Source: CAD feature listing. Evaluate the final solid. Frame: model axes, mm. Face numbers are marked on the shaded views. A direction names the side the tool comes from. Give positions to 0.01 mm unless a question says otherwise; leave off trailing zeros. Order: outer loops, then holes, each group sorted by start corner. A loop starts at its lowest first (then second) coordinate and runs counter-clockwise, first axis right, second up. Notation, with made-up numbers: (53, 41) - (87, 41) arc R10 ccw to (87, 58) - close; hole circle Ø3 at (2.5, 53.5). An arc over 180 degrees is marked (long way). Answer as CSV lines item,"result".
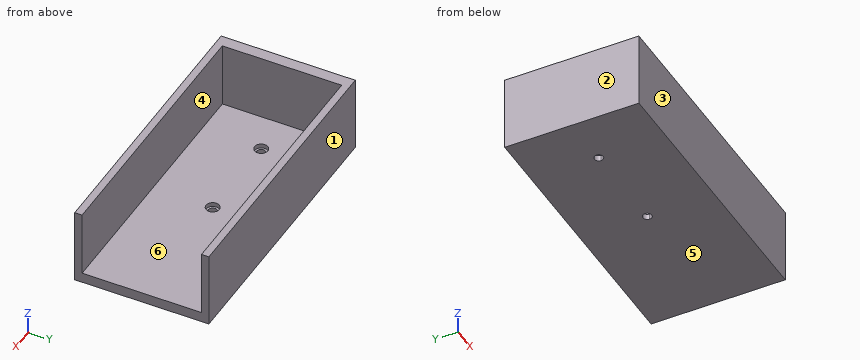
```python
from build123d import *

# Parameters (mm, degrees)
F1_DEPTH = 182
F2_W     = 91
F2_H     = 52
F3_DEPTH = 8
F5_DEPTH = 25
F6_R     = 4.5
F7_DEPTH = 3


with BuildPart() as f1:
    # F0 (on Right) → F1 (new body)
    with BuildSketch(Plane.YZ):
        Polygon((-0.5, -20), (-40.5, -20), (-40.5, 25), (-45.5, 25), (-45.5, -27), (45.5, -27), (45.5, 25), (40.5, 25), (40.5, -20), (0.5, -20), align=None)
    extrude(amount=F1_DEPTH)

    # F2 (on face) → F3 (join)
    with BuildSketch(Plane(origin=(0, 0, 0), x_dir=(0, -1, 0), z_dir=(-1, 0, 0))):
        with Locations((0, -1)):
            Rectangle(F2_W, F2_H)
    extrude(amount=F3_DEPTH)

    # F4 (on face) → F5 (cut)
    with BuildSketch(Plane.XY.offset(-20)):
        with BuildLine():
            ThreePointArc((30, 0), (29.12132, 2.12132), (27, 3))
            Line((27, 3), (27, -3))
            ThreePointArc((27, -3), (29.12132, -2.12132), (30, 0))
        make_face()
        with BuildLine():
            Line((27, -3), (27, 3))
            ThreePointArc((27, 3), (24, 0), (27, -3))
        make_face()
        with BuildLine():
            ThreePointArc((93, 0), (92.12132, 2.12132), (90, 3))
            Line((90, 3), (90, -3))
            ThreePointArc((90, -3), (92.12132, -2.12132), (93, 0))
        make_face()
        with BuildLine():
            Line((90, -3), (90, 3))
            ThreePointArc((90, 3), (87, 0), (90, -3))
        make_face()
    extrude(amount=-F5_DEPTH, mode=Mode.SUBTRACT)

    # F6 (on face) → F7 (cut)
    with BuildSketch(Plane.XY.offset(-20)):
        with Locations((27, 0)):
            Circle(F6_R)
        with Locations((90, 0)):
            Circle(F6_R)
    extrude(amount=-F7_DEPTH, mode=Mode.SUBTRACT)


solid = f1.part
```
(1) Cut plane A-A (x = 126). Return loops of the section in (y, z), then the cut area to 3 significant figures.
Completed:
outline,"(-45.5, -27) - (45.5, -27) - (45.5, 25) - (40.5, 25) - (40.5, -20) - (-40.5, -20) - (-40.5, 25) - (-45.5, 25) - close"
area,"1,090 mm²"
(2) Cut plane C-C (y = -10.5). Return loops of the section in (x, z).
Completed:
outline,"(-8, -27) - (182, -27) - (182, -20) - (0, -20) - (0, 25) - (-8, 25) - close"
(3) Mould query, pull axis Y, two halves, no side actions, for the marked faces 1, 2, 3 and 4. Classes: released by +Y, released by -Y, zero draft, split by the parting line, or undercut.
Completed:
face 1,"released by +Y"
face 2,"zero draft"
face 3,"released by -Y"
face 4,"undercut"
(4) Cut plane B-B (z = 4.5). Return loops of the section in (x, y).
Completed:
outline,"(-8, -45.5) - (182, -45.5) - (182, -40.5) - (0, -40.5) - (0, 40.5) - (182, 40.5) - (182, 45.5) - (-8, 45.5) - close"
(5) Access query for the marked faces 5 and 6. Directions: +Z, -Z, +X, -X, +Y, -Y. A direction counts if a zero-diameter tool reaches every point of the face in a straight line with its end or side. Return the directions, or none.
Completed:
face 5,"-Z, +X, -X, +Y, -Y"
face 6,"+Z, +X"
(6) Ray query, line 1 (Y direction, x = 46, z = -1.5); line 2 (X direction, y = 14.5, z = 15); line 3 (Z direction, x = 93, y = 1). Return the intervals inside material, ascending. Write a range as from..to.
Completed:
line 1,"-45.5..-40.5, 40.5..45.5"
line 2,"-8..0"
line 3,"-27..-23"
(7) Contact query for flat-ended pins moving along their axis: pin 1 (6 mm diameter, centred on y = 29, z = -16.5, fed in from +X); pin 2 (14.5 mm diameter, centred on x = 27, y = 0, fed in from +Z); pin 3 (2.5 mm diameter, centred on x = 28.5, y = 1, fed in from +Z). Output: stop coordinate, or through.
Completed:
pin 1,"x = 0"
pin 2,"z = -20"
pin 3,"z = -23"
